For this review, use the dimensioned drawing (mm, ordinates from the lowest corner) and the shaded views. A direction names the side the tool comes from. Give positions to 0.01 mm unless a question says otherwise; leave off trailing zeros. Loops run counter-clockwise (first coordinate to the right, second up) from the corner with the lowest first, then second, coordinate; pieces in that order, holes last. Notation, with made-up numbers: M -22,-2.75 L 4,-2.75 A29 ccw 4,33.25 Z; hole C 88,-15 d4. An arc over 180 degrees is marked long. Use a Markdown table: item, result. Add a question column.
(1) For the marked faces 1 and 2, list the 3-axis set-ups (+Z, -Z, +X, -X, +Y, -Y) from which the entire face can be reached by the end or side of a thin tool; tool diameter is ignored.
(2) Add section A-A, the plane x = 10. Give the boundary of the cut face in (y, z).
(3) For probe 1 along Y at (x, z) = (10, 1.6); probe 2 along Y at (x, z) = (10, 3.8), list the stretches that pass through material, from the lowest coordinate up.
(4) Add section D-D, the plane x = 3. Give the boundary of the cut face in (y, z), then the cut area to 3 significant figures.
(5) Add section C-C, the plane z = 0.3. Give the boundary of the cut face in (x, y).
(6) Draft analysis for pull direction X (two halves, no side actions). For the marked faces 3, 4 and 5, state which applies: pulls with the +X half, pulls with the -X half, needs draft (parallel to the pull), parting line crosses it, or undercut.
(7) Insertion check: pin 1 Ø3 at (x, y) = (2.5, 11) entering from +Z. The pin has a flat end and moves straight along its axis. Give the tip position at first contact, or say it passes through.
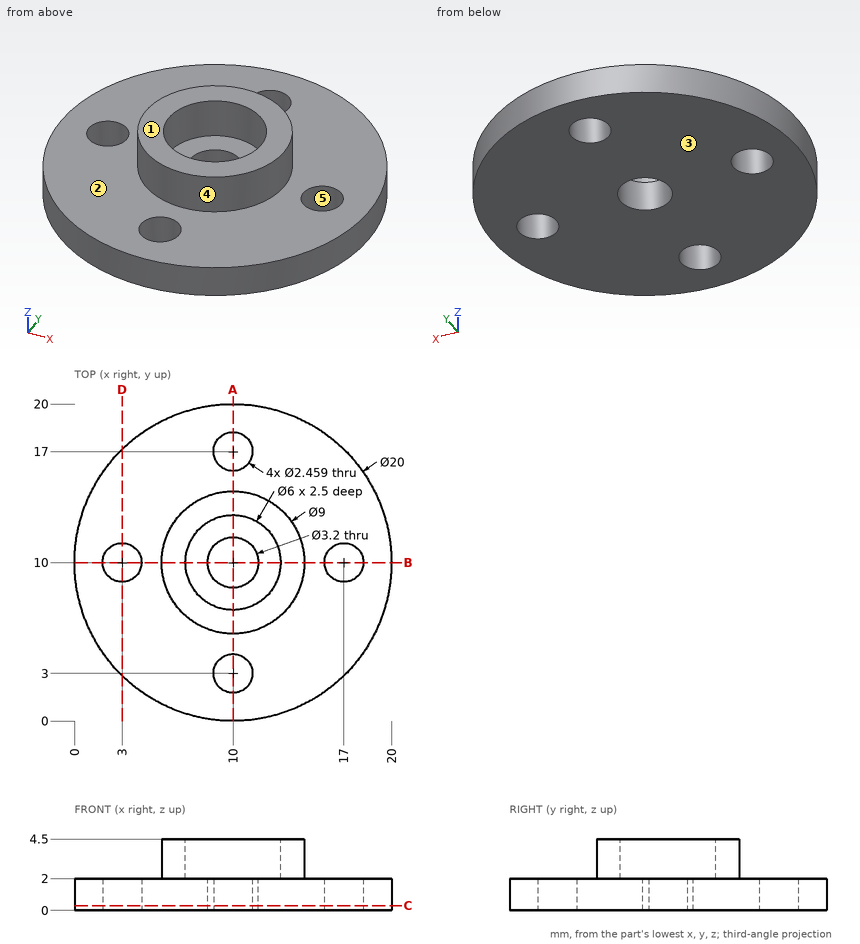
Established:
| question | item | result |
|---|---|---|
| 1 | face 1 | +Z, +X, -X, +Y, -Y |
| 1 | face 2 | +Z |
| 2 | outline | M 0,0 L 1.77,0 L 1.77,2 L 0,2 Z; M 4.23,0 L 8.4,0 L 8.4,2 L 7,2 L 7,4.5 L 5.5,4.5 L 5.5,2 L 4.23,2 Z; M 11.6,0 L 15.77,0 L 15.77,2 L 14.5,2 L 14.5,4.5 L 13,4.5 L 13,2 L 11.6,2 Z; M 18.23,0 L 20,0 L 20,2 L 18.23,2 Z |
| 3 | probe 1 | 0 to 1.77, 4.23 to 8.4, 11.6 to 15.77, 18.23 to 20 |
| 3 | probe 2 | 5.5 to 7, 13 to 14.5 |
| 4 | outline | M 2.86,0 L 8.77,0 L 8.77,2 L 2.86,2 Z; M 11.23,0 L 17.14,0 L 17.14,2 L 11.23,2 Z |
| 4 | area | 23.6 mm^2 |
| 5 | outline | C 10,10 d20; hole C 3,10 d2.46; hole C 10,10 d3.2; hole C 10,3 d2.46; hole C 10,17 d2.46; hole C 17,10 d2.46 |
| 6 | face 3 | needs draft |
| 6 | face 4 | parting line crosses it |
| 6 | face 5 | undercut |
| 7 | pin 1 | z = 2 |
